```python
from build123d import *

# Parameters (mm, degrees)
SKETCH1_W            = 35
SKETCH1_H            = 6.75
BOSS_EXTRUDE10_DEPTH = 3.5
SKETCH1_16_R         = 0.291434634
BOSS_EXTRUDE15_DEPTH = 1.25
SKETCH1_17_W         = 29
SKETCH1_17_H         = 2.924143722
BOSS_EXTRUDE17_DEPTH = 29.5
BOSS_EXTRUDE18_DEPTH = 1.25
SKETCH2_9_R          = 1.75
BOSS_EXTRUDE19_DEPTH = 1.75
FILLET1_R            = 2
FILLET2_R            = 4
SKETCH3_W            = 5.75
SKETCH3_H            = 0.795101344
CUT_EXTRUDE1_DEPTH   = 2.25


with BuildPart() as part:
    # Sketch1 → Boss-Extrude10 (new body)
    with BuildSketch(Plane.XY):
        with Locations((3, 3.375)):
            Rectangle(SKETCH1_W, SKETCH1_H)
        with BuildLine():
            Line((0, 6.25), (12.018477316, 5.016376067))
            ThreePointArc((12.018477316, 5.016376067), (13.5, 3.375), (12.018477316, 1.733623933))
            Line((12.018477316, 1.733623933), (0, 0.5))
            Line((0, 0.5), (-12.018477316, 1.733623933))
            ThreePointArc((-12.018477316, 1.733623933), (-13.5, 3.375), (-12.018477316, 5.016376067))
            Line((-12.018477316, 5.016376067), (0, 6.25))
        make_face(mode=Mode.SUBTRACT)
    extrude(amount=BOSS_EXTRUDE10_DEPTH)

    # Sketch1<16> → Boss-Extrude15 (add)
    # profile 1 of 9: a face of its own
    with BuildSketch(Plane.XY):
        with BuildLine():
            Line((-0.584049273, 6.190050878), (-12.018477316, 5.016376067))
            ThreePointArc((-12.018477316, 5.016376067), (-13.5, 3.375), (-12.018477316, 1.733623933))
            Line((-12.018477316, 1.733623933), (-0.584049273, 0.559949122))
            ThreePointArc((-0.584049273, 0.559949122), (-2.875, 3.375), (-0.584049273, 6.190050878))
        make_face()
        with Locations((-11.85, 3.375)):
            Circle(SKETCH1_16_R, mode=Mode.SUBTRACT)
        with Locations((-9.813185408, 3.375)):
            Circle(SKETCH1_16_R, mode=Mode.SUBTRACT)
        with Locations((-7.776370816, 3.375)):
            Circle(SKETCH1_16_R, mode=Mode.SUBTRACT)
    # profile 2 of 9: a face of its own
    with BuildSketch(Plane.XY):
        with Locations((-11.85, 3.375)):
            Circle(SKETCH1_16_R)
    # profile 3 of 9: a face of its own
    with BuildSketch(Plane.XY):
        with Locations((-7.776370816, 3.375)):
            Circle(SKETCH1_16_R)
    # profile 4 of 9: a face of its own
    with BuildSketch(Plane.XY):
        with Locations((-9.813185408, 3.375)):
            Circle(SKETCH1_16_R)
    # profile 5 of 9: a face of its own
    with BuildSketch(Plane.XY):
        with BuildLine():
            Line((0, 6.25), (-0.584049273, 6.190050878))
            ThreePointArc((-0.584049273, 6.190050878), (-2.875, 3.375), (-0.584049273, 0.559949122))
            Line((-0.584049273, 0.559949122), (0, 0.5))
            Line((0, 0.5), (0.584049273, 0.559949122))
            ThreePointArc((0.584049273, 0.559949122), (2.229884152, 1.56027091), (2.875, 3.375))
            ThreePointArc((2.875, 3.375), (2.229884152, 5.18972909), (0.584049273, 6.190050878))
            Line((0.584049273, 6.190050878), (0, 6.25))
        make_face()
    # profile 6 of 9: a face of its own
    with BuildSketch(Plane.XY):
        with BuildLine():
            Line((12.018477316, 5.016376067), (0.584049273, 6.190050878))
            ThreePointArc((0.584049273, 6.190050878), (2.229884152, 5.18972909), (2.875, 3.375))
            ThreePointArc((2.875, 3.375), (2.229884152, 1.56027091), (0.584049273, 0.559949122))
            Line((0.584049273, 0.559949122), (12.018477316, 1.733623933))
            ThreePointArc((12.018477316, 1.733623933), (13.5, 3.375), (12.018477316, 5.016376067))
        make_face()
        with Locations((7.776370816, 3.375)):
            Circle(SKETCH1_16_R, mode=Mode.SUBTRACT)
        with Locations((9.813185408, 3.375)):
            Circle(SKETCH1_16_R, mode=Mode.SUBTRACT)
        with Locations((11.85, 3.375)):
            Circle(SKETCH1_16_R, mode=Mode.SUBTRACT)
    # profile 7 of 9: a face of its own
    with BuildSketch(Plane.XY):
        with Locations((11.85, 3.375)):
            Circle(SKETCH1_16_R)
    # profile 8 of 9: a face of its own
    with BuildSketch(Plane.XY):
        with Locations((9.813185408, 3.375)):
            Circle(SKETCH1_16_R)
    # profile 9 of 9: a face of its own
    with BuildSketch(Plane.XY):
        with Locations((7.776370816, 3.375)):
            Circle(SKETCH1_16_R)
    extrude(amount=BOSS_EXTRUDE15_DEPTH)

    # Sketch1<17> → Boss-Extrude17 (add)
    with BuildSketch(Plane.XY):
        with Locations((35, 3.375)):
            Rectangle(SKETCH1_17_W, SKETCH1_17_H)
    extrude(amount=BOSS_EXTRUDE17_DEPTH)

    # Sketch2 → Boss-Extrude18 (add)
    with BuildSketch(Plane.XY.offset(29.5)):
        Polygon((14.5, 5.875), (-2.875, 5.875), (-2.875, 0.875), (14.5, 0.875), (20.5, 0.875), (20.5, 5.875), align=None)
    extrude(amount=-BOSS_EXTRUDE18_DEPTH)

    # Sketch2<9> → Boss-Extrude19 (add)
    with BuildSketch(Plane.XY.offset(29.5)):
        with Locations((0, 3.375)):
            Circle(SKETCH2_9_R)
    extrude(amount=BOSS_EXTRUDE19_DEPTH)

    # Fillet1
    # the kernel refuses this fillet: 2 mm, written as the material it adds along each edge
    with BuildSketch(Plane(origin=(20.5, 1.912928139, 0), x_dir=(0, -1, 0), z_dir=(0, 0, 1))) as fillet1_piece_1:
        with BuildLine():
            CenterArc((2, 1.998103724), FILLET1_R, 180, 87.504786267)
            Line((0, 1.998103724), (0, 0))
            Line((0, 0), (1.912928139, 0))
        make_face()
    extrude(amount=3.5)
    with BuildSketch(Plane(origin=(20.5, 4.837071861, 0), x_dir=(0, 1, 0), z_dir=(0, 0, 1))) as fillet1_piece_2:
        with BuildLine():
            CenterArc((2, -1.998103724), FILLET1_R, 92.495213733, 87.504786267)
            Line((0, -1.998103724), (0, 0))
            Line((0, 0), (1.912928139, 0))
        make_face()
    extrude(amount=3.5)
    with BuildSketch(Plane(origin=(20.5, 1.912928139, 28.25), x_dir=(1, 0, 0), z_dir=(0, 0, 1))) as fillet1_piece_3:
        with BuildLine():
            CenterArc((1.753401761, -2), FILLET1_R, 90, 61.246917848)
            Line((0, -1.037928139), (0, 0))
            Line((0, 0), (1.753401761, 0))
        make_face()
    extrude(amount=1.25)
    with BuildSketch(Plane(origin=(20.5, 4.837071861, 28.25), x_dir=(1, 0, 0), z_dir=(0, 0, 1))) as fillet1_piece_4:
        with BuildLine():
            CenterArc((1.753401761, 2), FILLET1_R, 208.753082152, 61.246917848)
            Line((0, 1.037928139), (0, 0))
            Line((0, 0), (1.753401761, 0))
        make_face()
    extrude(amount=1.25)

    # Fillet2
    # the kernel refuses this fillet: 4 mm, written as the material it takes off along each edge
    with BuildSketch(Plane(origin=(-14.5, 6.75, -10), x_dir=(0, -1, 0), z_dir=(0, 0, 1)), Plane(origin=(-14.5, 0, -10), x_dir=(1, 0, 0), z_dir=(0, 0, 1))) as fillet2_piece_1:
        with BuildLine():
            CenterArc((FILLET2_R, FILLET2_R), FILLET2_R, 180, 90)
            Line((0, FILLET2_R), (0, 0))
            Line((0, 0), (FILLET2_R, 0))
        make_face()
    extrude(amount=23.5, mode=Mode.SUBTRACT)

    # Sketch3 → Cut-Extrude1 (cut)
    with BuildSketch(Plane.XY.offset(3.5)):
        with Locations((0, 0.397550672)):
            Rectangle(SKETCH3_W, SKETCH3_H)
        with Locations((0, 6.352449328)):
            Rectangle(SKETCH3_W, SKETCH3_H)
    extrude(amount=-CUT_EXTRUDE1_DEPTH, mode=Mode.SUBTRACT)


solid = part.part
```
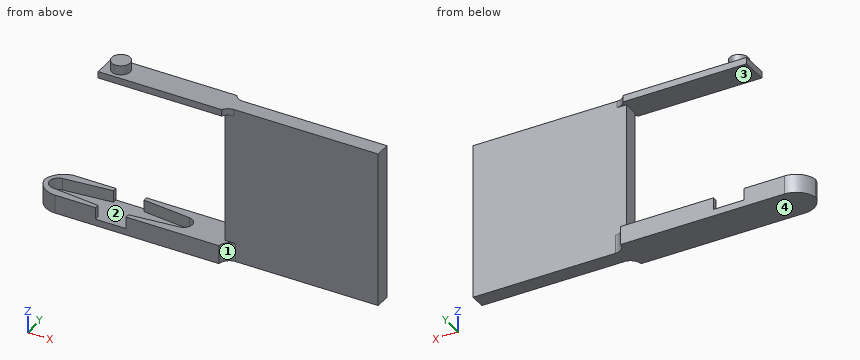
Check sheet for the modelled part. Datum: model origin and axes. Units: mm. Face numbers are marked on the shaded views. Round coordinates to 2 decimals unless told otherwise and drop trailing zeros. Order: outer loops, then holes, each group sorted by start corner. A loop starts at its lowest first (then second) coordinate and runs counter-clockwise, first axis right, second up. Notation, with made-up numbers: (-9.5, 58.25) - (27.5, 58.25) arc R12 ccw to (27.5, 71.25) - close; hole circle Ø4 at (82, 52). An arc over 180 degrees is marked (long way). Write item = value, one per line.
Q1. Draft check along Z on the marked faces 1, 2, 3 and 4. Enter one of: pulls with the +Z half, pulls with the -Z half, needs draft (parallel to the pull), parting line crosses it, or undercut.
Computed:
face_1 = needs draft
face_2 = undercut
face_3 = undercut
face_4 = pulls with the -Z half
Q2. Section check A-A (x = 0). Record the boundary of the cut face in (y, z) (3 decimals).
Computed:
outline = (0, 0) - (6.75, 0) - (6.75, 1.25) - (0, 1.25) - close; (0.875, 28.25) - (5.875, 28.25) - (5.875, 29.5) - (5.125, 29.5) - (5.125, 31.25) - (1.625, 31.25) - (1.625, 29.5) - (0.875, 29.5) - close
Q3. Section check D-D (x = 23.5). Record the boundary of the cut face in (y, z), and give its area (3 significant figures).
Computed:
outline = (1.91, 0) - (4.84, 0) - (4.84, 29.5) - (1.91, 29.5) - close
area = 86.3 mm^2
Q4. Thickness scan on line 1 along Z through (x, y) = (10, 1); line 2 along X through (y, z) = (3.25, 25); line 3 along Z through (x, y) = (23.5, 4.75). Record the ranges inside material, lowest first.
Computed:
line_1 = 0 to 3.5, 28.25 to 29.5
line_2 = 20.5 to 49.5
line_3 = 0 to 29.5
Q5. Go/stop test with flat-tipped pins: pin 1 (12 mm diameter, centred on x = -0.5, z = 24, fed in from -Y) (3 decimals); pin 2 (3 mm diameter, centred on y = 4, z = 15, fed in from -X); pin 3 (2 mm diameter, centred on x = -7.5, y = 5, fed in from +Z); pin 4 (12 mm diameter, centred on x = 6, z = 8.5, fed in from +Y). Record where each tip stops, or that it passes through.
Computed:
pin_1 = 0.875
pin_2 = 20.5
pin_3 = 3.5
pin_4 = 6.75
Q6. Section check B-B (y = 4). Record the boundary of the cut face in (x, z) (3 decimals), and give its area (3 significant figures).
Computed:
outline = (-14.3, 0) - (49.5, 0) - (49.5, 29.5) - (1.635, 29.5) - (1.635, 31.25) - (-1.635, 31.25) - (-1.635, 29.5) - (-2.875, 29.5) - (-2.875, 28.25) - (20.5, 28.25) - (20.5, 3.5) - (13.377, 3.5) - (13.377, 1.25) - (-13.377, 1.25) - (-13.377, 3.5) - (-14.3, 3.5) - close
area = 952 mm^2
Q7. Section check C-C (z = 25). Record the boundary of the cut face in (x, y), and give its area (3 significant figures).
Computed:
outline = (20.5, 1.91) - (49.5, 1.91) - (49.5, 4.84) - (20.5, 4.84) - close
area = 84.8 mm^2
